from build123d import *

# Parameters (mm, degrees)
F0_W      = 119.5
F0_H      = 22.5
F1_DEPTH  = 3
F3_D      = 8
F4_D      = 8
F5_W      = 8
F5_H      = 8.7
F6_DEPTH  = 3
F8_D      = 8
F9_D      = 8
F12_DEPTH = 3


with BuildPart() as f1:
    # F0 (on Front) → F1 (new body)
    with BuildSketch(Plane.XZ):
        Rectangle(F0_W, F0_H)
    extrude(amount=F1_DEPTH)

    # F3 (through all)
    with Locations(Plane.XZ.offset(3)):
        with Locations((-49.3088774383, 4.3802403379)):
            Hole(F3_D / 2)

    # F4 (through all)
    with Locations(Plane.XZ.offset(3)):
        with Locations((-49.35, -4.35)):
            Hole(F4_D / 2)

    # F5 (on face) → F6 (cut)
    with BuildSketch(Plane.XZ.offset(3)):
        with Locations((-49.3247925341, 0.0155190326)):
            Rectangle(F5_W, F5_H)
    extrude(amount=-F6_DEPTH, mode=Mode.SUBTRACT)

    # F8 (through all)
    with Locations(Plane.XZ.offset(3)):
        with Locations((49.35, 4.35)):
            Hole(F8_D / 2)

    # F9 (through all)
    with Locations(Plane.XZ.offset(3)):
        with Locations((49.35, -4.35)):
            Hole(F9_D / 2)

    # F11 (on face) → F12 (cut)
    with BuildSketch(Plane.XZ.offset(3)):
        Polygon((53.3259802461, -4.3563189382), (53.3259802461, 4.3436810618), (45.3259802461, 4.3436810618), (45.3259802461, -4.3563189382), (49.35, -4.3563189382), align=None)
    extrude(amount=-F12_DEPTH, mode=Mode.SUBTRACT)


solid = f1.part
Design review of the part built by this model. Coordinates are the model's own, in mm. A direction names the side the tool comes from. Give positions to 0.01 mm unless a question says otherwise; leave off trailing zeros. Order: outer loops, then holes, each group sorted by start corner. A loop starts at its lowest first (then second) coordinate and runs counter-clockwise, first axis right, second up. Notation, with made-up numbers: (61, -1.5) - (110, -1.5) arc R15 cw to (110, 8.5) - close; hole circle Ø2 at (-39.5, 14.5). An arc over 180 degrees is marked (long way). Write item = value, one per line. Start each with the question number.
Q1. Tool access review of faces 1 (the face through (-49.476, -1.479, -8.348)), 2 (the face through (59.75, -1, 0)): name each direction out of +Z, -Z, +X, -X, +Y, -Y from which nothing blocks a thin tool from reaching the whole face with its end or side.
Q2. We need section A-A on y = -1.6. State how many separate pieces and enclosed holes the cut face has, plus the area to 3 significant figures.
Q3. Mouldability with a two-part tool opening along Z and no side actions: class faces 3 (the face through (-53.325, -2, 0)), 4 (the face through (-1, -1, -11.25)), 5 (the face through (-1, 0, 0)) as released by +Z, released by -Z, zero draft, split by the parting line, or undercut.
Q4. We need section C-C on z = 1.5. State the section outline as (x, y) points.
Q5. To check wall thickness, follow L1, parallel to X at y = -1.6, z = -3.75; L2, parallel to X at y = -1.5, z = 8; L3, parallel to Z at x = 52, y = -2.2. State the ranges of each line that lie inside material, in increasing order. Write a range as from..to.
Q6. We need section D-D on x = -47. State the section outline as (y, z) points, plus the area to 3 significant figures.
Q7. We need section B-B on x = 49.35. State the section outline as (y, z) points.
Working result:
q1.face_1 = +Y, -Y
q1.face_2 = +Z, -Z, +X, +Y, -Y
q2.separate_pieces = 1
q2.enclosed_holes = 2
q2.area = 2,450 mm²
q3.face_3 = undercut
q3.face_4 = released by -Z
q3.face_5 = zero draft
q4.outline = (-59.75, -3) - (-53.32, -3) - (-53.32, 0) - (-59.75, 0) - close; (-45.32, -3) - (45.33, -3) - (45.33, 0) - (-45.32, 0) - close; (53.33, -3) - (59.75, -3) - (59.75, 0) - (53.33, 0) - close
q5.L1 = -59.75..-53.32, -45.32..45.33, 53.33..59.75
q5.L2 = -59.75..-51.01, -47.61..47.71, 50.99..59.75
q5.L3 = -11.25..-7.35, 7.35..11.25
q6.outline = (-3, -11.25) - (0, -11.25) - (0, -7.59) - (-3, -7.59) - close; (-3, 7.65) - (0, 7.65) - (0, 11.25) - (-3, 11.25) - close
q6.area = 21.8 mm²
q7.outline = (-3, -11.25) - (0, -11.25) - (0, -8.35) - (-3, -8.35) - close; (-3, 8.35) - (0, 8.35) - (0, 11.25) - (-3, 11.25) - close
